Job drawing, mm, ordinate dimensions from the low corner. One solid piece. Round coordinates to 2 decimals unless told otherwise and drop trailing zeros. Order: outer loops, then holes, each group sorted by start corner. A loop starts at its lowest first (then second) coordinate and runs counter-clockwise, first axis right, second up. Notation, with made-up numbers: (19, 78.5) -> (63, 78.5) arc R9 cw to (63, 92.5) -> close; hole circle Ø8 at (8, 31.5). An arc over 180 degrees is marked (long way). Answer as a JSON object with one key per item and string values. Group by question number.
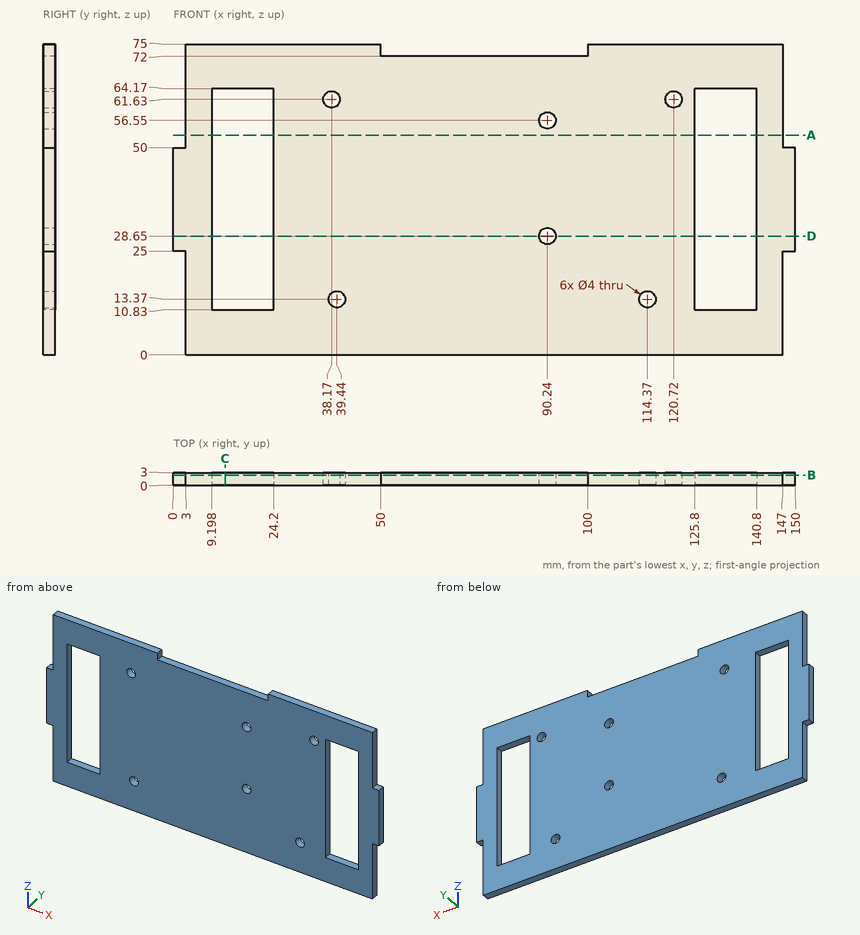
Q1. Drop flat-ended pins along their axis: pin 1 Ø4.5 at (x, z) = (90.24, 56.55) entering from -Y; pin 2 Ø1.5 at (y, z) = (1.5, 55) entering from +X; pin 3 Ø3.5 at (x, z) = (39.44, 13.37) entering from +Y; pin 4 Ø0.9 at (x, y) = (148.5, 1) entering from -Z. Give the stop position or say it passes through.
Q2. Band-saw the part on C-C (x = 12.5). List the corners of the cut face in (y, z).
Q3. Band-saw the part on A-A (z = 53). List the corners of the cut face in (x, y).
Q4. Band-saw the part on B-B (y = 2.45). Count the separate pieces of the cut face and the enclosed holes in it, plus the area to 3 significant figures.
Q5. Wall check: line 1 (X direction, y = 1.9, z = 61.63); line 2 (X direction, y = 1.55, z = 34.5); line 3 (X direction, y = 1.8, z = 13.37). Give the ranges that are in metal, low to high. Write a range as [from, to].
Q6. Band-saw the part on D-D (z = 28.65). List the corners of the cut face in (x, y), plus the area to 3 significant figures.
Completed:
{
 "1": {"pin 1": "y = 0", "pin 2": "x = 147", "pin 3": "through", "pin 4": "z = 25"},
 "2": {"outline": "(0, 0) -> (3, 0) -> (3, 10.83) -> (0, 10.83) -> close; (0, 64.17) -> (3, 64.17) -> (3, 75) -> (0, 75) -> close"},
 "3": {"outline": "(3, 0) -> (9.2, 0) -> (9.2, 3) -> (3, 3) -> close; (24.2, 0) -> (125.8, 0) -> (125.8, 3) -> (24.2, 3) -> close; (140.8, 0) -> (147, 0) -> (147, 3) -> (140.8, 3) -> close"},
 "4": {"separate pieces": "1", "enclosed holes": "8", "area": "9,120 mm2"},
 "5": {"line 1": "[3, 9.2], [24.2, 36.17], [40.17, 118.72], [122.72, 125.8], [140.8, 147]", "line 2": "[0, 9.2], [24.2, 125.8], [140.8, 150]", "line 3": "[3, 9.2], [24.2, 37.44], [41.44, 112.37], [116.37, 125.8], [140.8, 147]"},
 "6": {"outline": "(0, 0) -> (9.2, 0) -> (9.2, 3) -> (0, 3) -> close; (24.2, 0) -> (88.24, 0) -> (88.24, 3) -> (24.2, 3) -> close; (92.24, 0) -> (125.8, 0) -> (125.8, 3) -> (92.24, 3) -> close; (140.8, 0) -> (150, 0) -> (150, 3) -> (140.8, 3) -> close", "area": "348 mm2"}
}
